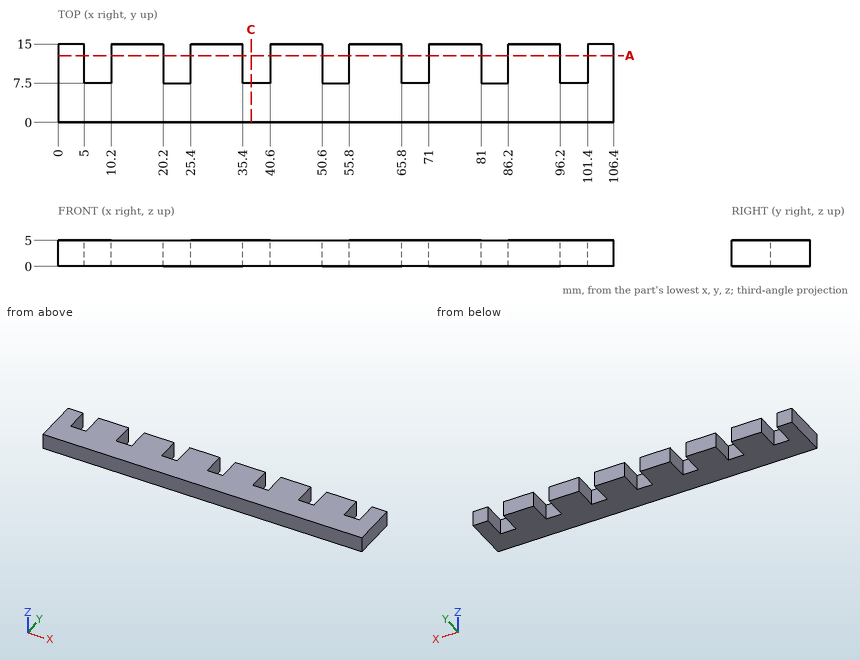
Can you work these out from the drawing? Everything is in mm from the part's minimum corner. Give positions to 0.01 mm unless a question says otherwise; leave off trailing zeros. Order: outer loops, then holes, each group sorted by start corner. A loop starts at its lowest first (then second) coordinate and runs counter-clockwise, first axis right, second up. Notation, with made-up numbers: (-37.5, -15.75) -> (9.5, -15.75) arc R18 cw to (9.5, 6.25) -> close; hole circle Ø11 at (15.5, -5.75). An arc over 180 degrees is marked (long way). Return JSON: item names as keys, results as strings.
1. Imagine slicing it at A-A on y = 12.75. Give the number of separate pieces and of enclosed holes in the cut face, then the cut area to 3 significant figures.
Answer list:
{"separate pieces": "8", "enclosed holes": "0", "area": "350 mm2"}
2. For pin 1 Ø1.5 at (x, z) = (69.5, 2) entering from +Y, with a flat end and sliding along its axis, tell me the tip position at first contact or that it passes through.
Answer list:
{"pin 1": "stops at y = 7.5"}
3. I need wall thicknesses on line 1 (Y direction, x = 10, z = 2.5). Which ranges of the line are inside material? Lowest first, please. Write a range as from..to.
Answer list:
{"line 1": "y = 0..7.5"}
4. Imagine slicing it at C-C on x = 37. List the corners of the cut face in (y, z) for me.
Answer list:
{"outline": "(0, 0) -> (7.5, 0) -> (7.5, 5) -> (0, 5) -> close"}
